Verification items for this drawing (mm, ordinates from the low corner). A direction names the side the tool comes from. Give positions to 0.01 mm unless a question says otherwise; leave off trailing zeros. Order: outer loops, then holes, each group sorted by start corner. A loop starts at its lowest first (then second) coordinate and runs counter-clockwise, first axis right, second up. Notation, with made-up numbers: M 85.25,-22.5 L 101.25,-22.5 A20 cw 101.25,7.5 Z; hole C 39.5,17 d7. An arc over 180 degrees is marked long. Answer as a JSON object with one key per item and string values.
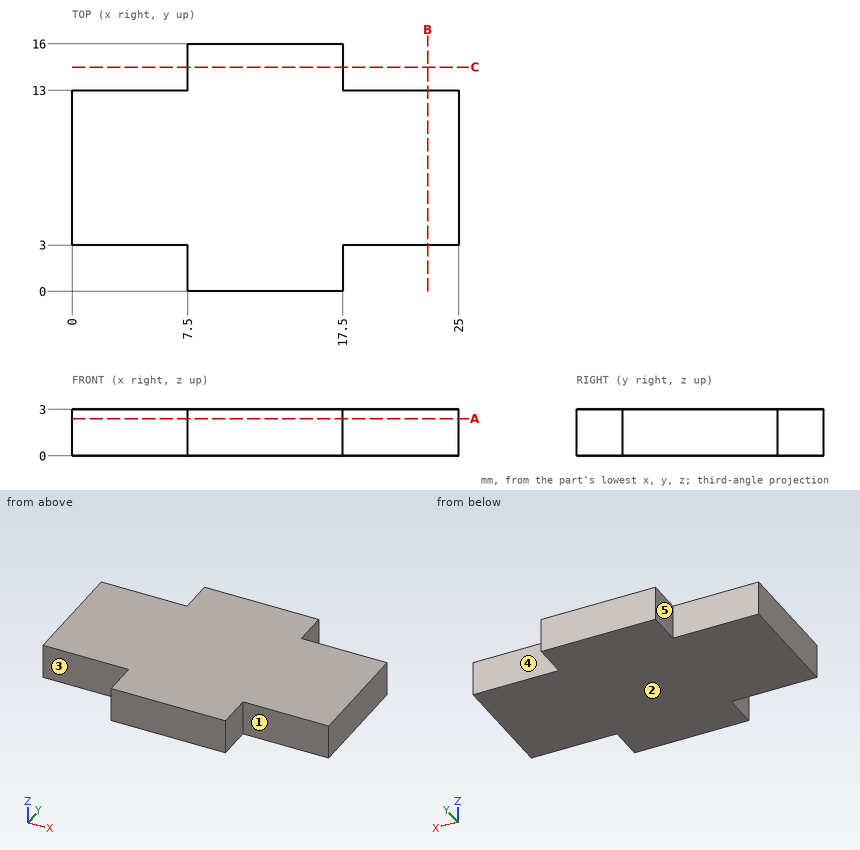
Q1. Tool access check on the marked faces 1, 2, 3, 4 and 5. Record the directions out of +Z, -Z, +X, -X, +Y, -Y that give a thin tool (end or side, any length) a straight path to the whole face; none if there is none.
Resolved:
{"face 1": "+Z, -Z, +X, -Y", "face 2": "-Z, +X, -X, +Y, -Y", "face 3": "+Z, -Z, -X, -Y", "face 4": "+Z, -Z, +X, +Y", "face 5": "+Z, -Z, -X, +Y"}
Q2. Gauge pin test, flat ends, axial feed: pin 1 Ø1.5 at (x, z) = (22.5, 1.5) entering from -Y; pin 2 Ø0.9 at (y, z) = (2, 1) entering from +X. Record the tip position at first contact, or that the pin passes through.
Resolved:
{"pin 1": "stops at y = 3", "pin 2": "stops at x = 17.5"}
Q3. Section check B-B on x = 23. Record the cut outline in (y, z), then the cut area to 3 significant figures.
Resolved:
{"outline": "M 3,0 L 13,0 L 13,3 L 3,3 Z", "area": "30.0 mm²"}
Q4. Section check A-A on z = 2.4. Record the cut outline in (x, y), then the cut area to 3 significant figures.
Resolved:
{"outline": "M 0,3 L 7.5,3 L 7.5,0 L 17.5,0 L 17.5,3 L 25,3 L 25,13 L 17.5,13 L 17.5,16 L 7.5,16 L 7.5,13 L 0,13 Z", "area": "310 mm²"}
Q5. Section check C-C on y = 14.5. Record the cut outline in (x, z).
Resolved:
{"outline": "M 7.5,0 L 17.5,0 L 17.5,3 L 7.5,3 Z"}
Q6. Material ranges on L1, parallel to Y at x = 22.5, z = 0.15; L2, parallel to X at y = 15, z = 0.4, recorded low to high.
Resolved:
{"L1": "y = 3 to 13", "L2": "x = 7.5 to 17.5"}
